Solid Edge part; units mm, degrees
sketch "Sketch1" plane through (0, 0, 0) normal (0, -1, 0) x (1, 0, 0)
  line L0 (8, 4.6188) -> (0, 9.2376)
  line L1 (0, 9.2376) -> (-8, 4.6188)
  line L2 (-8, 4.6188) -> (-8, -4.6188)
  line L3 (-8, -4.6188) -> (0, -9.2376)
  line L4 (0, -9.2376) -> (8, -4.6188)
  line L5 (8, -4.6188) -> (8, 4.6188)
extrude "Protrusion1" add sketch "Sketch1" along normal mid plane 9
sketch "Sketch2" plane through (0, 0, 0) normal (1, 0, 0) x (0, 1, 0)
  line L0 (-4.5, 7.315) -> (-3.9848, 9.2376)
revolve "RevolvedCutout1" cut sketch "Sketch2" angle 360 about axis through (0, 0, 0) along (0, -1, 0) material side at (0, -4.2907, 8.2892)
hole "孔_7" at (0, -4.5, 0) direction (0, 1, 0) diameter 8.376 end up to next start chamfer 1 start chamfer angle 60 end chamfer 1 end chamfer angle 60
sketch "Sketch3" plane through (0, 0, 0) normal (1, 0, 0) x (0, 1, 0)
  line L0 (4.5, -7.4905) -> (1.4739, -9.2376)
revolve "RevolvedCutout2" cut sketch "Sketch3" angle 360 about axis through (0, 0, 0) along (0, 1, 0) material side at (0, 3.0119, -8.4074)
The model under review builds one solid part; all positions refer to its coordinate system, in mm. Round coordinates to 2 decimals unless told otherwise and drop trailing zeros. Write each loop counter-clockwise with the first axis right and the second up, starting at its lowest first coordinate (ties: lowest second). Pieces come first, ordered by that corner, then holes. Notation, with made-up numbers: M -23.5,60 L 31.5,60 A30 cw 31.5,89 Z; hole C -12.5,12.25 d4. An arc over 180 degrees is marked long. Use a Markdown table: item, result. Add a question column.
Q1. We need section B-B, the plane y = -2.75. State the section outline as (x, z) points.
Q2. To check wall thickness, follow line 1 (X direction, y = 1.5, z = 0); line 2 (Z direction, x = 2, y = -3); line 3 (Z direction, x = 1.5, y = 2). State the ranges of each line that lie inside material, in increasing order.
Q3. Insertion check: pin 1 (6.5 mm diameter, centred on x = 0, z = 0, fed in from -Y); pin 2 (4 mm diameter, centred on x = 3, y = 2, fed in from +Z). Each pin has a flat end and moves straight along its axis. Give the tip position at first contact, or say it passes through.
Q4. We need section A-A, the plane z = 0. State the section outline as (x, y) points (1 decimal).
Q5. We need section C-C, the plane y = 2.75. State the section outline as (x, z) points.
Q6. The part is to be moulded in two halves that separate along X. For faces 1 (the face through (-4.056, -0.294, -6.896)), 2 (the face through (-5, 4.5, 2)), 3 (the face through (2.83, -0.055, 3.087)), 4 (the face through (4.056, -0.294, 6.896)), say which applies: pulls with the +X half, pulls with the -X half, needs draft (parallel to the pull), parting line crosses it, or undercut.
Findings below:
| question | item | result |
|---|---|---|
| 1 | outline | M -8,-4.62 L 0,-9.24 L 8,-4.62 L 8,4.62 L 0,9.24 L -8,4.62 Z; hole C 0,0 d8.38 |
| 2 | line 1 | x = -8 to -4.19, 4.19 to 8 |
| 2 | line 2 | z = -8.08 to -3.68, 3.68 to 8.08 |
| 2 | line 3 | z = -8.37 to -3.91, 3.91 to 8.37 |
| 3 | pin 1 | passes through |
| 3 | pin 2 | stops at z = 8.66 |
| 4 | outline | M -8,-4.3 L -7.3,-4.5 L -5.2,-4.5 L -4.2,-3.9 L -4.2,3.9 L -5.2,4.5 L -7.5,4.5 L -8,3.6 Z; M 4.2,-3.9 L 5.2,-4.5 L 7.3,-4.5 L 8,-4.3 L 8,3.6 L 7.5,4.5 L 5.2,4.5 L 4.2,3.9 Z |
| 5 | outline | M -8,-2.87 A8.5 ccw -6.49,-5.49 L -1.51,-8.37 A8.5 ccw 1.51,-8.37 L 6.49,-5.49 A8.5 ccw 8,-2.87 L 8,2.87 A8.5 ccw 6.49,5.49 L 1.51,8.37 A8.5 ccw -1.51,8.37 L -6.49,5.49 A8.5 ccw -8,2.87 Z; hole C 0,0 d8.38 |
| 6 | face 1 | pulls with the -X half |
| 6 | face 2 | needs draft |
| 6 | face 3 | undercut |
| 6 | face 4 | pulls with the +X half |
